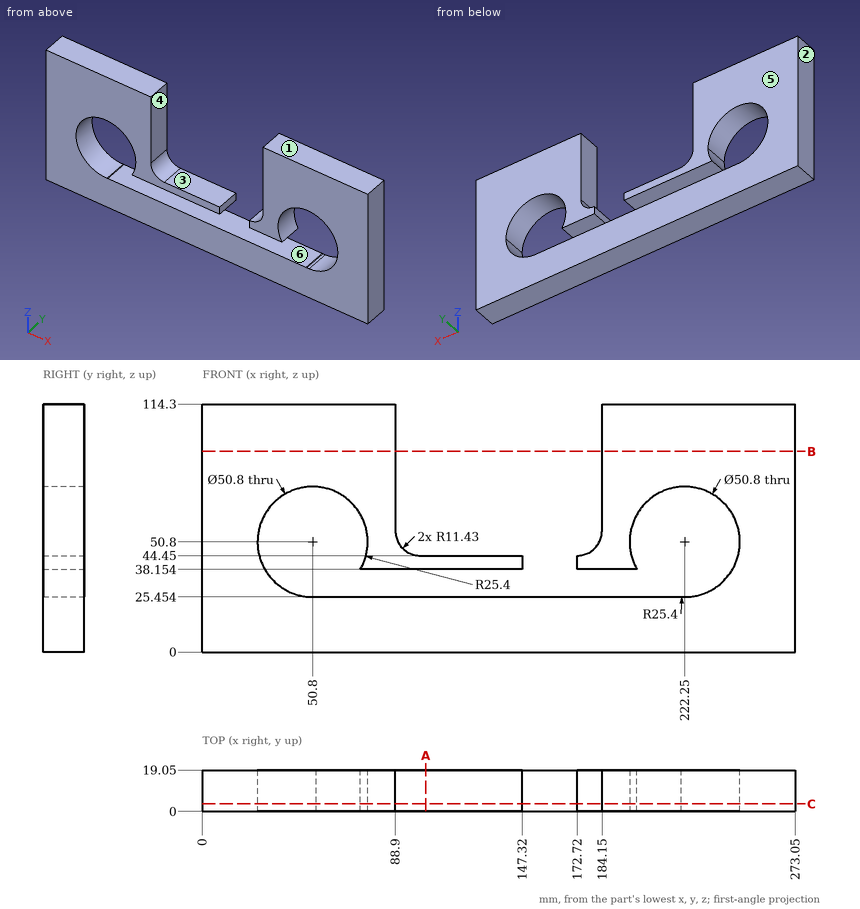
Source: three-view drawing plus pictorial views. Frame: mm from the lowest corner of the part. A direction names the side the tool comes from. Round coordinates to 2 decimals unless told otherwise and drop trailing zeros. Loops run counter-clockwise (first coordinate to the right, second up) from the corner with the lowest first, then second, coordinate; pieces in that order, holes last.
Q1. Access query for the marked faces 4, 5 and 6. Directions: +Z, -Z, +X, -X, +Y, -Y. A direction counts if a zero-diameter tool reaches every point of the face in a straight line with its end or side. Return the directions, or none.
Q2. Pull-direction query (X, two-part tool) for the marked faces 1, 2 and 3; classes: released by +X, released by -X, zero draft, split by the parting line, or undercut.
Q3. Section A-A on x = 103. Return loops of the section in (y, z).
Q4. Material intervals for L1, parallel to Z at x = 222.25, y = 8.5; L2, parallel to X at y = 7.25, z = 50.8; L3, parallel to X at y = 5.25, z = 100, sorted ascending.
Q5. Section C-C on y = 3.5. Return loops of the section in (x, z).
Q6. Section B-B on z = 92.5. Return loops of the section in (x, y), plus the area to 3 significant figures.
Evaluation:
1. face 4: +Z, +Y, -Y
1. face 5: +Z, -Z, +X, -X, +Y
1. face 6: +Y, -Y
2. face 1: zero draft
2. face 2: released by -X
2. face 3: undercut
3. outline: (0, 0) - (19.05, 0) - (19.05, 25.45) - (0, 25.45) - close; (0, 38.15) - (19.05, 38.15) - (19.05, 44.45) - (0, 44.45) - close
4. L1: z = 0 to 25.4, 76.2 to 114.3
4. L2: x = 0 to 25.4, 76.2 to 90.09, 182.96 to 196.85, 247.65 to 273.05
4. L3: x = 0 to 88.9, 184.15 to 273.05
5. outline: (0, 0) - (273.05, 0) - (273.05, 114.3) - (184.15, 114.3) - (184.15, 55.88) arc R11.43 cw to (172.72, 44.45) - (172.72, 38.15) - (200.22, 38.15) arc R25.4 cw (long way) to (220.59, 25.45) - (52.46, 25.45) arc R25.4 cw (long way) to (72.83, 38.15) - (147.32, 38.15) - (147.32, 44.45) - (100.33, 44.45) arc R11.43 cw to (88.9, 55.88) - (88.9, 114.3) - (0, 114.3) - close
6. outline: (0, 0) - (88.9, 0) - (88.9, 19.05) - (0, 19.05) - close; (184.15, 0) - (273.05, 0) - (273.05, 19.05) - (184.15, 19.05) - close
6. area: 3,390 mm2
